Source: three-view drawing plus pictorial views. Frame: mm from the lowest corner of the part. Round coordinates to 2 decimals unless told otherwise and drop trailing zeros. Write each loop counter-clockwise with the first axis right and the second up, starting at its lowest first coordinate (ties: lowest second). Pieces come first, ordered by that corner, then holes. Notation, with made-up numbers: M 41.5,21.25 L 88.5,21.25 A35 cw 88.5,54.25 Z; hole C 71.25,10.25 d10. An arc over 180 degrees is marked long. Answer as CSV lines item,"result". Start each with the question number.
Q1. Section query B-B on y = 39.5. Output: boundary loops of the cut face in (x, z) (1 decimal).
Q2. Section query A-A on z = 1.4. Output: boundary loops of the cut face in (x, y) (1 decimal).
Q3. Section query C-C on x = 65. Output: boundary loops of the cut face in (y, z) (1 decimal).
Q4. Ray query, probe 1 along Y at (x, z) = (181, 0.45) (1 decimal); probe 2 along X at (y, z) = (176, 1.2) (1 decimal). Return the intervals inside material, ascending.
Q5. First-contact query: pin 1 (1 mm diameter, centred on x = 217, z = 2, fed in from +Y) (1 decimal); pin 2 (1.6 mm diameter, centred on y = 2, z = 2.5, fed in from -X); pin 3 (1 mm diameter, centred on y = 160.5, z = 2, fed in from -X) (1 decimal); pin 4 (1 mm diameter, centred on x = 124, z = 1.5, fed in from -Y). Flat tips, straight axial feed; report the tip coordinate or a pass-through.
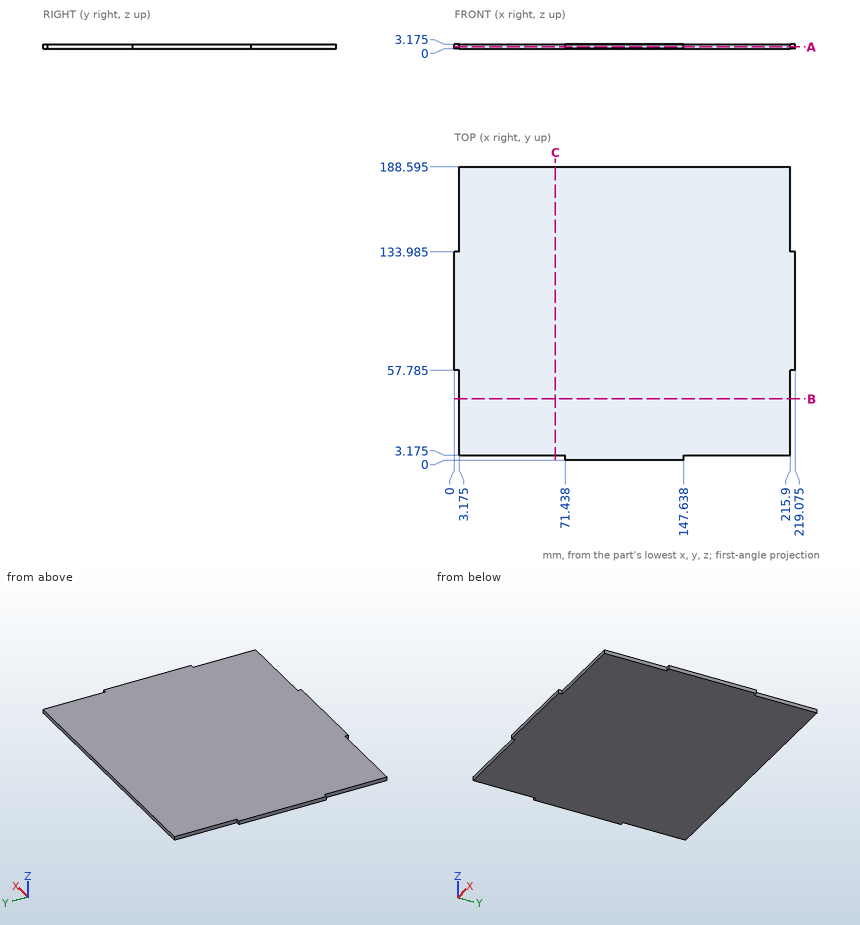
Entries:
1,outline,"M 3.2,0 L 215.9,0 L 215.9,3.2 L 3.2,3.2 Z"
2,outline,"M 0,57.8 L 3.2,57.8 L 3.2,3.2 L 71.4,3.2 L 71.4,0 L 147.6,0 L 147.6,3.2 L 215.9,3.2 L 215.9,57.8 L 219.1,57.8 L 219.1,134 L 215.9,134 L 215.9,188.6 L 3.2,188.6 L 3.2,134 L 0,134 Z"
3,outline,"M 3.2,0 L 188.6,0 L 188.6,3.2 L 3.2,3.2 Z"
4,probe 1,"y = 3.2 to 188.6"
4,probe 2,"x = 3.2 to 215.9"
5,pin 1,"stops at y = 134"
5,pin 2,"stops at x = 71.44"
5,pin 3,"stops at x = 3.2"
5,pin 4,"stops at y = 0"
